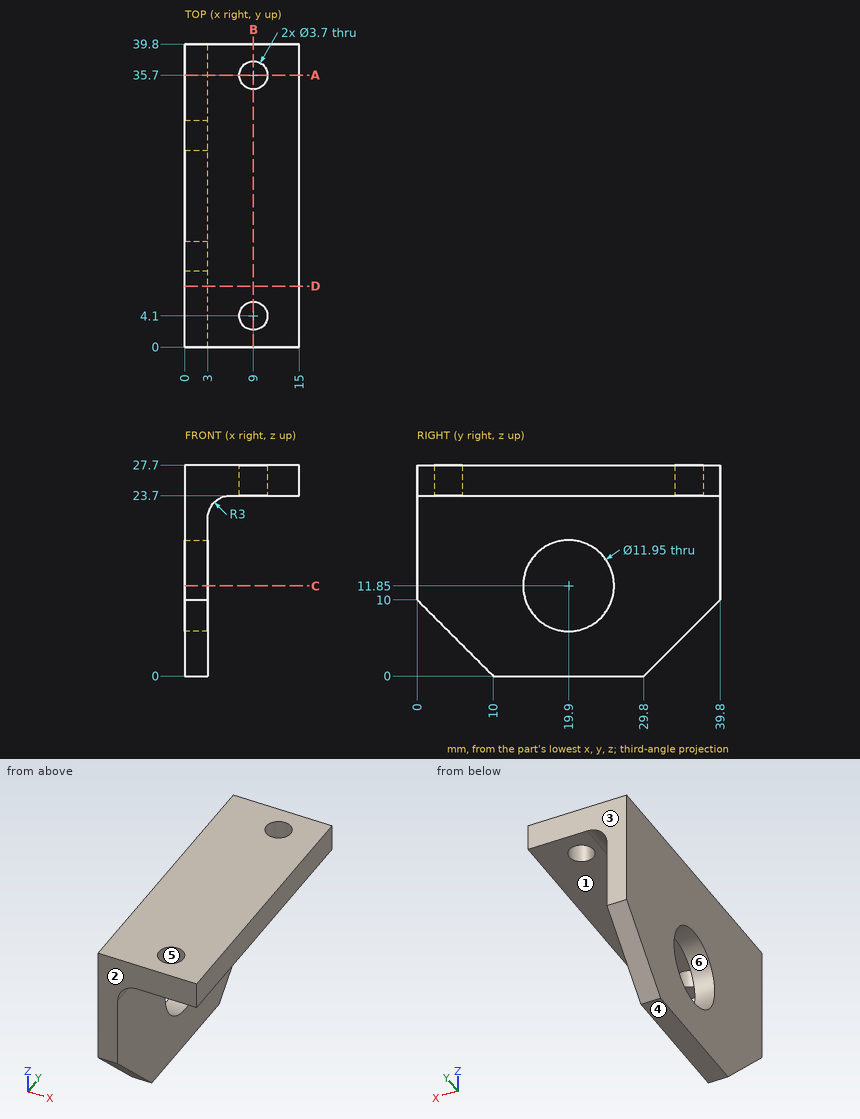
Answer from the drawing. Dimensions are ordinates in mm from the lowest x, y and z of the part. A direction names the side the tool comes from. Coordinates: 2 decimals unless noted, no trailing zeros. Write each loop counter-clockwise with the first axis right and the second up, starting at its lowest first coordinate (ties: lowest second). Pieces come first, ordered by that corner, then holes. Notation, with made-up numbers: M 2.5,28.25 L 28.5,28.25 A27 cw 28.5,46.25 Z; hole C -33,76 d2. An arc over 180 degrees is marked long. Use one line per item in the form item = value. Start each with the question number.
1. Each of these flat-tipped pins is pushed along its axis until it touches: P1, Ø4, axis at x = 8.5, y = 35.5, coming from the -Z side; P2, Ø6, axis at x = 7.5, y = 28.5, coming from the -Z side; P3, Ø10.5, axis at y = 27, z = 7.5, coming from the +X side. Where does it stop, or does it pass through?
2. The part is cut by section A-A (y = 35.7). Give the vertices of the cut face in (x, z).
3. The mould has two halves that part along Y. Classify the marked faces 3, 4, 5 and 6: released by +Y, released by -Y, zero draft, split by the parting line, or undercut.
4. The part is cut by section D-D (y = 8). Give the vertices of the cut face in (x, z).
5. The part is cut by section C-C (z = 11.85). Give the vertices of the cut face in (x, y) (3 decimals), plus the area to 4 significant figures.
6. A tool of negligible diameter and unlimited length cuts with its end or side. For the marked faces 1 and 2, from which of +Z, -Z, +X, -X, +Y, -Y can it reach the whole face along a straight path? Write none if from no direction.
7. The part is cut by section B-B (x = 9). Give the vertices of the cut face in (y, z), plus the area to 3 significant figures.
8. Straight lines are drawn through the part: probe 1 along Y at (x, z) = (1.5, 11.85) (3 decimals); probe 2 along X at (y, z) = (28.5, 16.5); probe 3 along Z at (x, y) = (12.75, 14.5). For each, find the intervals that lie inside material, in ascending order. Write a range as from..to.
Evaluation:
q1.P1 = 23.7
q1.P2 = 23.3
q1.P3 = 3
q2.outline = M 0,5.9 L 3,5.9 L 3,20.7 A3 cw 6,23.7 L 7.15,23.7 L 7.15,27.7 L 0,27.7 Z; M 10.85,23.7 L 15,23.7 L 15,27.7 L 10.85,27.7 Z
q3.face_3 = released by +Y
q3.face_4 = zero draft
q3.face_5 = undercut
q3.face_6 = undercut
q4.outline = M 0,2 L 3,2 L 3,20.7 A3 cw 6,23.7 L 15,23.7 L 15,27.7 L 0,27.7 Z
q5.outline = M 0,0 L 3,0 L 3,13.925 L 0,13.925 Z; M 0,25.875 L 3,25.875 L 3,39.8 L 0,39.8 Z
q5.area = 83.55 mm^2
q6.face_1 = -Z, +X, +Y, -Y
q6.face_2 = +Z, -Z, +X, -X, -Y
q7.outline = M 0,23.7 L 2.25,23.7 L 2.25,27.7 L 0,27.7 Z; M 5.95,23.7 L 33.85,23.7 L 33.85,27.7 L 5.95,27.7 Z; M 37.55,23.7 L 39.8,23.7 L 39.8,27.7 L 37.55,27.7 Z
q7.area = 130 mm^2
q8.probe_1 = 0..13.925, 25.875..39.8
q8.probe_2 = 0..3
q8.probe_3 = 23.7..27.7
